Read the model definition and answer for the solid it produces. Units are mm, in the model's axes. Coordinates: 2 decimals unless noted, no trailing zeros. Order: outer loops, then holes, each group sorted by start corner. A loop starts at its lowest first (then second) coordinate and runs counter-clockwise, first axis right, second up. Notation, with made-up numbers: (38.25, 31.25) -> (84.25, 31.25) arc R29 ccw to (84.25, 58.25) -> close; hole circle Ø6 at (2, 35). An arc over 180 degrees is marked (long way). Answer as a JSON object with one key per item and string values. Group by question number.
1) Section C-C on y = 89 is taken. Determine the outline of the cut face in (x, z) (3 decimals), and give its area (3 significant figures).
2) Section A-A on x = 0 is taken. Determine the outline of the cut face in (y, z) (3 decimals).
3) Given pin 1 (1 mm diameter, centred on x = 1.5, y = 25, fed in from +Z), flat-ended and moving along its own axis, determine where the tip first touches the part or whether it passes through.
4) Consider L1, parallel to X at y = 18.5, z = 0.25; L2, parallel to Y at x = -2.25, z = -0.25; L3, parallel to Z at x = -2.25, y = 12. Determine where each line is inside the solid, lowest interval first.
5) Section B-B on y = 43 is taken. Determine the outline of the cut face in (x, z) (3 decimals), and give its area (3 significant figures).
from build123d import *

# Parameters (mm, degrees)
SKETCH1_R               = 3.175
BOSS_EXTRUDE1_DEPTH     = 97
CUT_EXTRUDE1_DEPTH      = 98.103868358
CUT_EXTRUDE1_DEPTH_BACK = 21


with BuildPart() as part:
    # Sketch1 → Boss-Extrude1 (new body)
    with BuildSketch(Plane(origin=(0, 0, 0), x_dir=(1, 0, 0), z_dir=(0, 1, 0))):
        with Locations(Location((0, 0, 0), (0, 0, 90))):
            Circle(SKETCH1_R)
    extrude(amount=BOSS_EXTRUDE1_DEPTH)

    # Sketch2 → Cut-Extrude1 (cut, two sides: drawn at the far end of the back side and taken through both)
    with BuildSketch(Plane(origin=(0, 97, 0), x_dir=(1, 0, 0), z_dir=(0, 1, 0)).offset(-CUT_EXTRUDE1_DEPTH_BACK)):
        Polygon((-26.82080565, 2.517016971), (-1.610698227, 2.736106032), (1.562902146, 2.763686285), (26.773009569, 2.982775346), (26.334831446, 53.402990191), (-27.258983772, 52.937231816), align=None)
    extrude(amount=CUT_EXTRUDE1_DEPTH + CUT_EXTRUDE1_DEPTH_BACK, mode=Mode.SUBTRACT)

    # Fillet1: read off the stored shape, not the designer's step
    # Fillet1 outline → Fillet1 (revolve, cut)
    with BuildSketch(Plane.XY):
        with BuildLine():
            ThreePointArc((3.175, 1), (2.882106781, 0.292893219), (2.175, 0))
            Line((2.175, 0), (3.175, 0))
            Line((3.175, 0), (3.175, 1))
        make_face()
        with BuildLine():
            ThreePointArc((2.175, 97), (2.882106781, 96.707106781), (3.175, 96))
            Line((3.175, 96), (3.175, 97))
            Line((3.175, 97), (2.175, 97))
        make_face()
    revolve(axis=Axis((0, 0, 0), (0, 1, 0)), mode=Mode.SUBTRACT)


solid = part.part
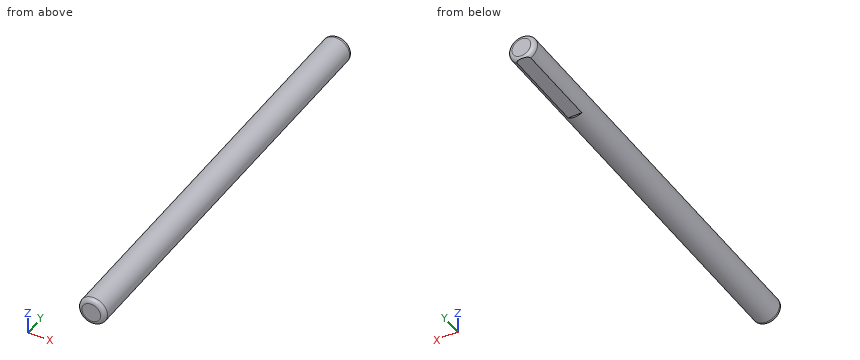
Worked answers:
{
 "1": {"outline": "(-1.611, -2.736) -> (1.563, -2.764) arc R3.175 ccw (long way) to start", "area": "30.8 mm²"},
 "2": {"outline": "(0, -2.175) arc R1 ccw to (1, -3.175) -> (76, -3.175) -> (76, -2.75) -> (96.818, -2.75) arc R1 ccw to (97, -2.175) -> (97, 2.175) arc R1 ccw to (96, 3.175) -> (1, 3.175) arc R1 ccw to (0, 2.175) -> close"},
 "3": {"pin 1": "stops at z = 3.01"},
 "4": {"L1": "x = -3.17 to 3.17", "L2": "y = 0 to 97", "L3": "z = -2.24 to 2.24"},
 "5": {"outline": "circle Ø6.35 at (0, 0)", "area": "31.7 mm²"}
}
